For this review, use the dimensioned drawing (mm, ordinates from the lowest corner) and the shaded views. A direction names the side the tool comes from. Round coordinates to 2 decimals unless told otherwise and drop trailing zeros. Loops run counter-clockwise (first coordinate to the right, second up) from the corner with the lowest first, then second, coordinate; pieces in that order, holes last. Notation, with made-up numbers: (88, 54) - (141, 54) arc R23 cw to (141, 86) - close; hole circle Ø10 at (-13.75, 70). An arc over 180 degrees is marked (long way). One line per question, with ' | ' between items. Start each with the question number.
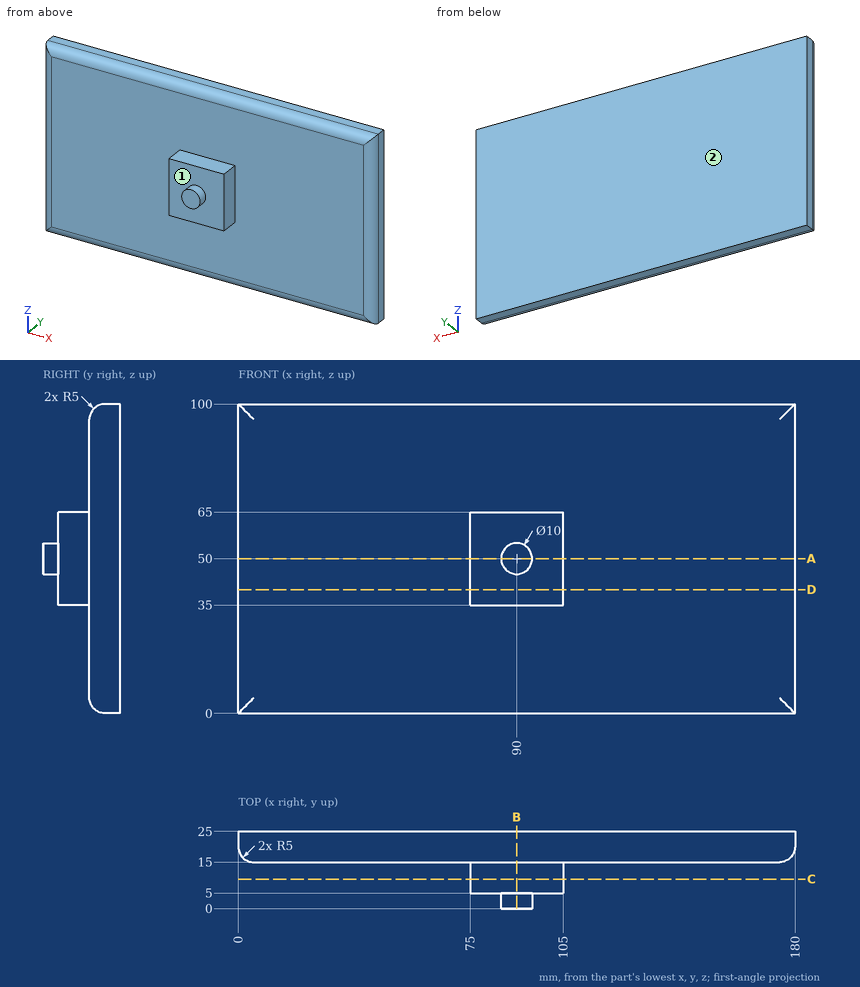
1. Take a section at C-C, the plane y = 9.5. Give the boundary of the cut face in (x, z), then the cut area to 3 significant figures.
2. Clearance check with flat-ended pins moving along their axes: P1, Ø8, axis at x = 103, y = 3, coming from the +Z side; P2, Ø2, axis at x = 145, y = 16.5, coming from the -Z side; P3, Ø12, axis at x = 46, z = 48, coming from the -Y side. State where each tip first meets the part, or that it passes through.
3. Take a section at A-A, the plane z = 50. Give the boundary of the cut face in (x, y).
4. Take a section at B-B, the plane x = 90. Give the boundary of the cut face in (y, z), then the cut area to 3 significant figures.
5. Take a section at D-D, the plane z = 40. Give the boundary of the cut face in (x, y).
6. To check wall thickness, follow line 1 along Y through (x, z) = (164.5, 76); line 2 along X through (y, z) = (12, 58); line 3 along Y through (x, z) = (104.5, 40). State the ranges of each line that lie inside material, in increasing order.
7. Machinability: for the marked faces 1 and 2, which of the approach directions +Z, -Z, +X, -X, +Y, -Y give a long, thin tool a straight path to every point of the face, cutting with its end or side? Answer none if there is none.
Answer list:
1) outline: (75, 35) - (105, 35) - (105, 65) - (75, 65) - close | area: 900 mm²
2) P1: stops at z = 65 | P2: stops at z = 0.67 | P3: stops at y = 15
3) outline: (0, 20) arc R5 ccw to (5, 15) - (75, 15) - (75, 5) - (85, 5) - (85, 0) - (95, 0) - (95, 5) - (105, 5) - (105, 15) - (175, 15) arc R5 ccw to (180, 20) - (180, 25) - (0, 25) - close
4) outline: (0, 45) - (5, 45) - (5, 35) - (15, 35) - (15, 5) arc R5 ccw to (20, 0) - (25, 0) - (25, 100) - (20, 100) arc R5 ccw to (15, 95) - (15, 65) - (5, 65) - (5, 55) - (0, 55) - close | area: 1,340 mm²
5) outline: (0, 20) arc R5 ccw to (5, 15) - (75, 15) - (75, 5) - (105, 5) - (105, 15) - (175, 15) arc R5 ccw to (180, 20) - (180, 25) - (0, 25) - close
6) line 1: y = 15 to 25 | line 2: x = 75 to 105 | line 3: y = 5 to 25
7) face 1: -Y | face 2: +Z, -Z, +X, -X, +Y
